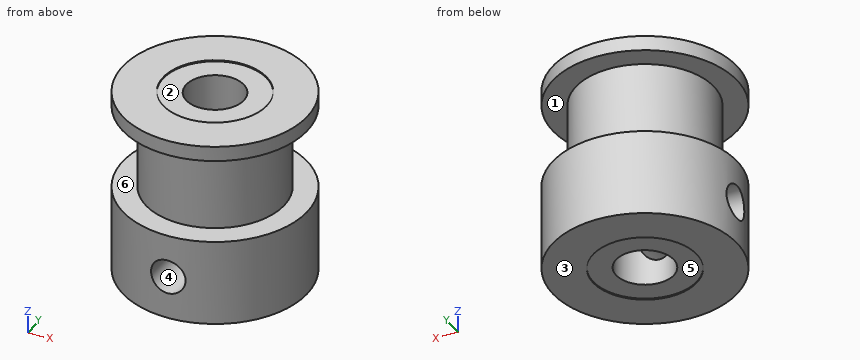
```python
from build123d import *

# Parameters (mm, degrees)
SKETCH1_R           = 8
BOSS_EXTRUDE1_DEPTH = 7.5
SKETCH2_R           = 6
BOSS_EXTRUDE2_DEPTH = 7.4
SKETCH3_R           = 8
BOSS_EXTRUDE3_DEPTH = 1.3
SKETCH4_R           = 2.5
CUT_EXTRUDE1_DEPTH  = 20
SKETCH5_R           = 4.5
CUT_EXTRUDE2_DEPTH  = 0.1
CUT_EXTRUDE3_START  = -0.1
SKETCH6_R           = 4.5
CUT_EXTRUDE3_DEPTH  = 0.1
SKETCH7_R           = 1.5
CUT_EXTRUDE4_DEPTH  = 20
SKETCH8_R           = 1.5
CUT_EXTRUDE5_DEPTH  = 20


with BuildPart() as part:
    # Sketch1 → Boss-Extrude1 (new body)
    with BuildSketch(Plane.XY):
        Circle(SKETCH1_R)
    extrude(amount=BOSS_EXTRUDE1_DEPTH)

    # Sketch2 → Boss-Extrude2 (add)
    with BuildSketch(Plane.XY.offset(7.5)):
        Circle(SKETCH2_R)
    extrude(amount=BOSS_EXTRUDE2_DEPTH)

    # Sketch3 → Boss-Extrude3 (add)
    with BuildSketch(Plane.XY.offset(14.9)):
        Circle(SKETCH3_R)
    extrude(amount=BOSS_EXTRUDE3_DEPTH)

    # Sketch4 → Cut-Extrude1 (cut)
    with BuildSketch(Plane.XY.offset(16.2)):
        Circle(SKETCH4_R)
    extrude(amount=-CUT_EXTRUDE1_DEPTH, mode=Mode.SUBTRACT)

    # Sketch5 → Cut-Extrude2 (cut)
    with BuildSketch(Plane.XY.offset(16.2)):
        Circle(SKETCH5_R)
    extrude(amount=-CUT_EXTRUDE2_DEPTH, mode=Mode.SUBTRACT)

    # Sketch6 → Cut-Extrude3 (cut)
    with BuildSketch(Plane(origin=(0, 0, 0), x_dir=(-1, 0, 0), z_dir=(0, 0, -1)).offset(CUT_EXTRUDE3_START)):
        with Locations(Location((0, 0, 0), (0, 0, 180))):
            Circle(SKETCH6_R)
    extrude(amount=CUT_EXTRUDE3_DEPTH, mode=Mode.SUBTRACT)

    # Sketch7 → Cut-Extrude4 (cut)
    with BuildSketch(Plane(origin=(0, 0, 0), x_dir=(0, 0, -1), z_dir=(1, 0, 0))):
        with Locations((-3.75, 0)):
            Circle(SKETCH7_R)
    extrude(amount=-CUT_EXTRUDE4_DEPTH, mode=Mode.SUBTRACT)

    # Sketch8 → Cut-Extrude5 (cut)
    with BuildSketch(Plane(origin=(0, 0, 0), x_dir=(1, 0, 0), z_dir=(0, 1, 0))):
        with Locations(Location((0, -3.75, 0), (0, 0, 270))):
            Circle(SKETCH8_R)
    extrude(amount=-CUT_EXTRUDE5_DEPTH, mode=Mode.SUBTRACT)


solid = part.part
```
Here's how the part is built. I have some questions about the finished solid (model axes, mm). Face numbers are marked on the shaded views. A direction names the side the tool comes from. Coordinates: 2 decimals unless noted, no trailing zeros. Order: outer loops, then holes, each group sorted by start corner. A loop starts at its lowest first (then second) coordinate and runs counter-clockwise, first axis right, second up.
1) Imagine slicing it at C-C on z = 3.5. List the corners of the cut face in (x, y) for me, and give its area (3 significant figures).
2) We'd pull the mould along Z, two halves only. Please class the marked faces 1, 2 and 3: +Z half, -Z half, draft (parallel to the pull), parting line (faces both ways), or undercut.
3) Imagine slicing it at A-A on x = 0. List the corners of the cut face in (y, z) for me, and give its area (3 significant figures).
4) I need wall thicknesses on line 1 (Z direction, x = 6.75, y = -2.25); line 2 (Z direction, x = 0, y = -3.5); line 3 (X direction, y = 0.5, z = 8.75). Which ranges of each line are inside material? Lowest first, please.
5) Will these pins go through, and if not, where does the flat tip stop? pin 1 (3 mm diameter, centred on x = 2.5, z = 11.5, fed in from -Y); pin 2 (1 mm diameter, centred on x = 2.5, z = 4, fed in from -Y); pin 3 (5 mm diameter, centred on y = -2, z = 9.5, fed in from -X); pin 4 (1 mm diameter, centred on x = -0.5, y = -6, fed in from -Z).
6) Imagine slicing it at D-D on x = -4.75. List the corners of the cut face in (y, z) for me.
7) Which directions (+Z, -Z, +X, -X, +Y, -Y) give clear straight access to the entire face, cutting with the end or side of a thin tool? Please do the marked faces 4, 5 and 6.
Response values:
1. outline: (-7.86, -1.48) arc R8 ccw to (-1.48, -7.86) - (-1.48, -2.02) arc R2.5 cw to (-2.02, -1.48) - close; (-7.86, 1.48) - (-2.02, 1.48) arc R2.5 cw (long way) to (1.48, -2.02) - (1.48, -7.86) arc R8 ccw (long way) to start
1. area: 148 mm2
2. face 1: undercut
2. face 2: +Z half
2. face 3: -Z half
3. outline: (-8, 0) - (-4.5, 0) - (-4.5, 0.1) - (-2.5, 0.1) - (-2.5, 2.25) - (-8, 2.25) - close; (-8, 5.25) - (-2.5, 5.25) - (-2.5, 16.1) - (-4.5, 16.1) - (-4.5, 16.2) - (-8, 16.2) - (-8, 14.9) - (-6, 14.9) - (-6, 7.5) - (-8, 7.5) - close; (2.5, 0.1) - (4.5, 0.1) - (4.5, 0) - (8, 0) - (8, 7.5) - (6, 7.5) - (6, 14.9) - (8, 14.9) - (8, 16.2) - (4.5, 16.2) - (4.5, 16.1) - (2.5, 16.1) - close
3. area: 131 mm2
4. line 1: z = 0 to 7.5, 14.9 to 16.2
4. line 2: z = 0.1 to 2.25, 5.25 to 16.1
4. line 3: x = -5.98 to -2.45, 2.45 to 5.98
5. pin 1: stops at y = -5.92
5. pin 2: stops at y = -7.75
5. pin 3: stops at x = -7.98
5. pin 4: stops at z = 0
6. outline: (-6.44, 0) - (6.44, 0) - (6.44, 7.5) - (3.67, 7.5) - (3.67, 14.9) - (6.44, 14.9) - (6.44, 16.2) - (-6.44, 16.2) - (-6.44, 14.9) - (-3.67, 14.9) - (-3.67, 7.5) - (-6.44, 7.5) - close; hole circle Ø3 at (0, 3.75)
7. face 4: -Y
7. face 5: -Z
7. face 6: none
